from build123d import *

# Parameters (mm, degrees)
F1_DEPTH = 609.6
F2_R     = 9.525
F2_R_2   = 2.38125
F2_R_3   = 6.35
F3_DEPTH = 50.801
F4_R     = 2.38125
F5_DEPTH = 3.175
F6_R     = 4.7625
F6_R_2   = 6.35
F6_R_3   = 8.73125
F6_R_4   = 2.38125
F7_DEPTH = 3.175


with BuildPart() as f1:
    # F0 (on Front) → F1 (new body)
    with BuildSketch(Plane.XZ):
        Polygon((-27.920566, 91.871106), (-27.920566, 79.171106), (-24.745566, 79.171106), (-24.745566, 88.696106), (19.704434, 88.696106), (19.704434, -85.928894), (22.879434, -85.928894), (22.879434, 91.871106), align=None)
    extrude(amount=F1_DEPTH)

    # F2 (on face) → F3 (cut, through all)
    with BuildSketch(Plane.YZ.offset(22.879434)):
        with Locations((-435.76875, 41.071106)):
            Circle(F2_R)
        with Locations((-365.91875, 41.071106)):
            Circle(F2_R)
        with Locations((-296.06875, 41.071106)):
            Circle(F2_R)
        with Locations((-226.21875, 41.071106)):
            Circle(F2_R)
        with Locations((-156.36875, 41.071106)):
            Circle(F2_R)
        with Locations((-603.25, -73.228894)):
            Circle(F2_R_2)
        with Locations((-547.6875, -73.228894)):
            Circle(F2_R_3)
        with Locations((-490.5375, -73.228894)):
            Circle(F2_R_3)
        with Locations((-361.95, -73.228894)):
            Circle(F2_R_3)
        with Locations((-444.5, -73.228894)):
            Circle(F2_R_2)
        with Locations((-304.8, -73.228894)):
            Circle(F2_R_2)
        with Locations((-247.65, -73.228894)):
            Circle(F2_R_3)
        with Locations((-165.1, -73.228894)):
            Circle(F2_R_2)
        with Locations((-109.5375, -73.228894)):
            Circle(F2_R_3)
        with Locations((-52.3875, -73.228894)):
            Circle(F2_R_3)
        with Locations((-6.35, -73.228894)):
            Circle(F2_R_2)
    extrude(amount=-F3_DEPTH, mode=Mode.SUBTRACT)

    # F4 (on face) → F5 (cut, through all)
    with BuildSketch(Plane(origin=(-27.920566, 0, 0), x_dir=(0, -1, 0), z_dir=(-1, 0, 0))):
        with Locations((6.35, 85.521106)):
            Circle(F4_R)
        with Locations((165.1, 85.521106)):
            Circle(F4_R)
        with Locations((304.8, 85.521106)):
            Circle(F4_R)
        with Locations((444.5, 85.521106)):
            Circle(F4_R)
        with Locations((603.25, 85.521106)):
            Circle(F4_R)
    extrude(amount=-F5_DEPTH, mode=Mode.SUBTRACT)

    # F6 (on face) → F7 (cut, through all)
    with BuildSketch(Plane.XY.offset(91.871106)):
        with Locations((10.179434, -60.325)):
            Circle(F6_R)
        with Locations((-15.220566, -60.325)):
            Circle(F6_R)
        with Locations((10.179434, -95.25)):
            Circle(F6_R)
        with Locations((-15.220566, -95.25)):
            Circle(F6_R)
        with Locations((-2.520566, -133.35)):
            Circle(F6_R)
        with Locations((-2.520566, -179.3875)):
            Circle(F6_R)
        with Locations((-2.520566, -225.425)):
            Circle(F6_R)
        with Locations((-2.520566, -317.5)):
            Circle(F6_R)
        with Locations((-2.520566, -409.575)):
            Circle(F6_R)
        with Locations((-2.520566, -501.65)):
            Circle(F6_R_2)
        with Locations((-2.520566, -363.5375)):
            Circle(F6_R)
        with Locations((-2.520566, -271.4625)):
            Circle(F6_R)
        with Locations((-2.520566, -523.875)):
            Circle(F6_R_2)
        with Locations((-2.520566, -549.275)):
            Circle(F6_R_3)
        with Locations((-2.520566, -455.6125)):
            Circle(F6_R)
        with Locations((-2.520566, -6.35)):
            Circle(F6_R_4)
        with Locations((-2.520566, -603.25)):
            Circle(F6_R_4)
    extrude(amount=-F7_DEPTH, mode=Mode.SUBTRACT)


solid = f1.part
The listing builds one solid part. Answer for the finished solid, in the listing's coordinates (mm). A direction names the side the tool comes from. Round coordinates to 2 decimals unless told otherwise and drop trailing zeros. Order: outer loops, then holes, each group sorted by start corner. A loop starts at its lowest first (then second) coordinate and runs counter-clockwise, first axis right, second up. Notation, with made-up numbers: (63, -3.75) -> (69, -3.75) arc R23 cw to (69, 29.25) -> close; hole circle Ø4 at (49, 15). An arc over 180 degrees is marked (long way). Write each question's results on one line, items separated by ' | '. Start each with the question number.
Q1. Find section C-C (z = -8). Determine the outline of the cut face in (x, y), then the cut area to 3 significant figures.
Q2. Each of these flat-tipped pins is pushed along its axis until it touches: pin 1 (1.5 mm diameter, centred on x = 17, y = -396, fed in from -Z); pin 2 (4.5 mm diameter, centred on y = -603.25, z = 85.52, fed in from -X); pin 3 (7.5 mm diameter, centred on y = -547.69, z = -73.23, fed in from -X); pin 4 (1.6 mm diameter, centred on x = -26, y = -269.5, fed in from -Z). Where does it stop, or does it pass through?
Q3. Straight lines are drawn through the part: probe 1 along Z at (x, y) = (-26.75, -444.5); probe 2 along Z at (x, y) = (15.5, -170); probe 3 along X at (y, z) = (-341.5, 66). For each, find the intervals that lie inside material, in ascending order. Write a range as from..to.
Q4. Find section B-B (y = -80). Determine the outline of the cut face in (x, z).
Q5. The mould has two halves that part along Y. Classify faces 3 (the flat face through (20, 0, 30)), 4 (the flat face through (-3, -301, 88.696)), 5 (the cylindrical face through (-3.897, -530.074, 90.306)), 6 (the cylindrical face through (21.31, -115.88, -72.95)): pulls with the +Y half, pulls with the -Y half, needs draft (parallel to the pull), parting line crosses it, or undercut.
Q6. Which of the six approach directions +Z, -Z, +X, -X, +Y, -Y give full straight-line access (tool end or side, diameter ignored) to faces 1 (the cylindrical face through (21.31, -46.33, -71.32)), 2 (the flat face through (19.704, -301, 3))?
Q7. Find section A-A (y = -247.65). Determine the outline of the cut face in (x, z).
Worked answers:
1) outline: (19.7, -609.6) -> (22.88, -609.6) -> (22.88, 0) -> (19.7, 0) -> close | area: 1,940 mm2
2) pin 1: stops at z = 88.7 | pin 2: stops at x = 19.7 | pin 3: passes through | pin 4: stops at z = 79.17
3) probe 1: z = 79.17..83.14, 87.9..91.87 | probe 2: z = 88.7..91.87 | probe 3: x = 19.7..22.88
4) outline: (-27.92, 79.17) -> (-24.75, 79.17) -> (-24.75, 88.7) -> (19.7, 88.7) -> (19.7, -85.93) -> (22.88, -85.93) -> (22.88, 91.87) -> (-27.92, 91.87) -> close
5) face 3: pulls with the +Y half | face 4: needs draft | face 5: undercut | face 6: undercut
6) face 1: +X, -X | face 2: -Z, +Y, -Y
7) outline: (-27.92, 79.17) -> (-24.75, 79.17) -> (-24.75, 88.7) -> (19.7, 88.7) -> (19.7, -66.88) -> (22.88, -66.88) -> (22.88, 91.87) -> (-27.92, 91.87) -> close; (19.7, -85.93) -> (22.88, -85.93) -> (22.88, -79.58) -> (19.7, -79.58) -> close
